Geometry: see drawing. Coordinates: mm, zero at the bounding-box minimum. A direction names the side the tool comes from. Coordinates: 2 decimals unless noted, no trailing zeros. Order: outer loops, then holes, each group sorted by start corner. A loop starts at its lowest first (then second) coordinate and runs counter-clockwise, first axis right, second up. Notation, with made-up numbers: (-33, 89) -> (-21, 89) arc R18 ccw to (-21, 106) -> close; hole circle Ø9 at (1.25, -23). An arc over 180 degrees is marked (long way). Use one line per item in the form item = value.
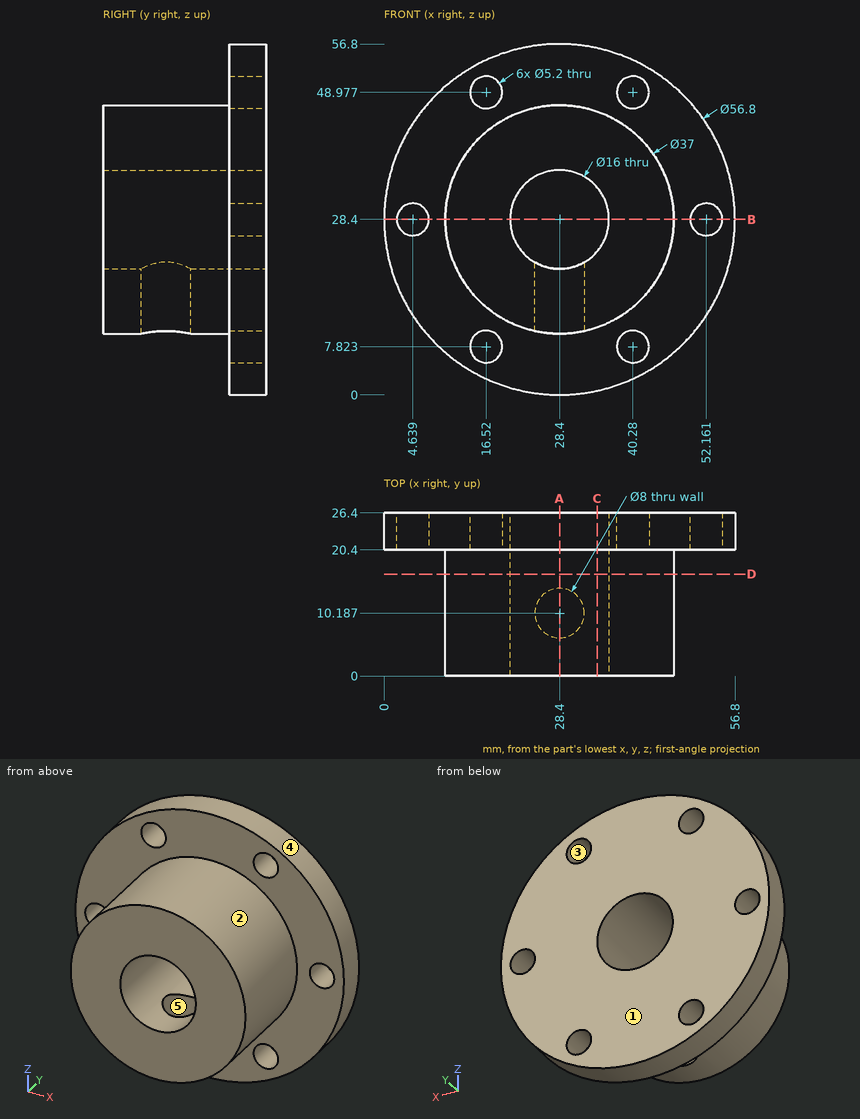
1) Section D-D, the plane y = 16.5. Output: boundary loops of the cut face in (x, z), and give its area (3 significant figures).
Results found:
outline = circle Ø37 at (28.4, 28.4); hole circle Ø16 at (28.4, 28.4)
area = 874 mm2
2) Section B-B, the plane z = 28.4. Output: boundary loops of the cut face in (x, y), and give its area (3 significant figures).
Results found:
outline = (0, 20.4) -> (2.04, 20.4) -> (2.04, 26.4) -> (0, 26.4) -> close; (7.24, 20.4) -> (9.9, 20.4) -> (9.9, 0) -> (20.4, 0) -> (20.4, 26.4) -> (7.24, 26.4) -> close; (36.4, 0) -> (46.9, 0) -> (46.9, 20.4) -> (49.56, 20.4) -> (49.56, 26.4) -> (36.4, 26.4) -> close; (54.76, 20.4) -> (56.8, 20.4) -> (56.8, 26.4) -> (54.76, 26.4) -> close
area = 611 mm2
3) Section A-A, the plane x = 28.4. Output: boundary loops of the cut face in (y, z), and give its area (3 significant figures).
Results found:
outline = (0, 9.9) -> (6.19, 9.9) -> (6.19, 20.4) -> (0, 20.4) -> close; (0, 36.4) -> (26.4, 36.4) -> (26.4, 56.8) -> (20.4, 56.8) -> (20.4, 46.9) -> (0, 46.9) -> close; (14.19, 9.9) -> (20.4, 9.9) -> (20.4, 0) -> (26.4, 0) -> (26.4, 20.4) -> (14.19, 20.4) -> close
area = 589 mm2
4) Pull-direction query (Z, two-part tool) for the marked faces 3, 4 and 5; classes: released by +Z, released by -Z, zero draft, split by the parting line, or undercut.
Results found:
face_3 = undercut
face_4 = split by the parting line
face_5 = zero draft
5) Section C-C, the plane x = 34.5. Output: boundary loops of the cut face in (y, z) (1 decimal), and give its area (3 significant figures).
Results found:
outline = (0, 10.9) -> (20.4, 10.9) -> (20.4, 0.7) -> (26.4, 0.7) -> (26.4, 23.2) -> (0, 23.2) -> close; (0, 33.6) -> (26.4, 33.6) -> (26.4, 56.1) -> (20.4, 56.1) -> (20.4, 45.9) -> (0, 45.9) -> close
area = 772 mm2
6) Material intervals for probe 1 along Z at (x, y) = (28.4, 19.5); probe 2 along Y at (x, z) = (28.4, 14.75); probe 3 along Y at (x, z) = (43.5, 49.5), sorted ascending. Write a range as from..to.
Results found:
probe_1 = 9.9..20.4, 36.4..46.9
probe_2 = 0..6.19, 14.19..26.4
probe_3 = 20.4..26.4
7) Contact query for flat-ended pins moving along their axis: P1, Ø10, axis at x = 15, y = 3.5, coming from the +Z side; P2, Ø8, axis at y = 20, z = 18, coming from the -X side (1 decimal); P3, Ø8.5, axis at x = 40.28, z = 48.98, coming from the -Y side; P4, Ø6, axis at x = 52.16, z = 28.4, coming from the +Y side. Output: stop coordinate, or through.
Results found:
P1 = 44.88
P2 = 0.7
P3 = 20.4
P4 = 26.4
8) Access query for the marked faces 1 and 2. Directions: +Z, -Z, +X, -X, +Y, -Y. A direction counts if a zero-diameter tool reaches every point of the face in a straight line with its end or side. Return the directions, or none.
Results found:
face_1 = +Z, -Z, +X, -X, +Y
face_2 = -Y
